```python
from build123d import *

# Parameters (mm, degrees)
BOSS_EXTRUDE1_DEPTH = 163.1
SKETCH3_W           = 29.8
SKETCH3_H           = 11.8
BOSS_EXTRUDE2_DEPTH = 4.2


with BuildPart() as part:
    # Sketch2 → Boss-Extrude1 (new body)
    with BuildSketch(Plane.XY):
        Polygon((42.7, 0), (-42.7, 0), (-42.7, 2.2), (-45.7, 2.2), (-45.7, 4.2), (45.7, 4.2), (45.7, 2.2), (42.7, 2.2), align=None)
    extrude(amount=BOSS_EXTRUDE1_DEPTH)

    # Sketch3 → Boss-Extrude2 (add)
    with BuildSketch(Plane.XZ):
        with Locations((0, 169)):
            Rectangle(SKETCH3_W, SKETCH3_H)
    extrude(amount=-BOSS_EXTRUDE2_DEPTH)


solid = part.part
```
Could you check a few things on this model? Use its own coordinates, in mm. A direction names the side the tool comes from. Round coordinates to 2 decimals unless told otherwise and drop trailing zeros. Order: outer loops, then holes, each group sorted by start corner. A loop starts at its lowest first (then second) coordinate and runs counter-clockwise, first axis right, second up. Notation, with made-up numbers: M -33,7.25 L -13,7.25 A10 cw -13,21.25 Z; hole C -19,-20.5 d9. An arc over 180 degrees is marked long. One line per question, with ' | ' between items. Start each with the question number.
(1) For P1, Ø3.5, axis at x = -44.5, z = 54.5, coming from the -Y side; P2, Ø1.3, axis at x = -37.5, y = 2.5, coming from the +Z side; P3, Ø2.5, axis at y = 0.5, z = 50.5, coming from the -X side, each with a flat end and sliding along its axis, tell me the tip position at first contact or that it passes through.
(2) Suppose I cut it at C-C on x = 17. List the corners of the cut face in (y, z) for me, then the cut area to 3 significant figures.
(3) Please list where these lines run through material, in increasing order: line 1 along Z through (x, y) = (-17, 1.55); line 2 along X through (y, z) = (0.8, 100).
(4) For faces 1 (the face through (-30, 2, 163.1)), 2 (the face through (44, 2.2, 80)), 3 (the face through (-44, 2.2, 80)), which set-ups out of +Z, -Z, +X, -X, +Y, -Y let a thin tool reach every point of the face, with its end or its side?
(5) Suppose I cut it at B-B on z = 150. List the corners of the cut face in (x, y) for me, then the cut area to 3 significant figures.
(6) Suppose I cut it at A-A on y = 1.25. List the corners of the cut face in (x, z) for me, then the cut area to 3 significant figures.
Geometry results:
1) P1: y = 2.2 | P2: z = 163.1 | P3: x = -42.7
2) outline: M 0,0 L 4.2,0 L 4.2,163.1 L 0,163.1 Z | area: 685 mm²
3) line 1: 0 to 163.1 | line 2: -42.7 to 42.7
4) face 1: +Z, -X, +Y, -Y | face 2: +Z, -Z, +X, -Y | face 3: +Z, -Z, -X, -Y
5) outline: M -45.7,2.2 L -42.7,2.2 L -42.7,0 L 42.7,0 L 42.7,2.2 L 45.7,2.2 L 45.7,4.2 L -45.7,4.2 Z | area: 371 mm²
6) outline: M -42.7,0 L 42.7,0 L 42.7,163.1 L 14.9,163.1 L 14.9,174.9 L -14.9,174.9 L -14.9,163.1 L -42.7,163.1 Z | area: 14,300 mm²
